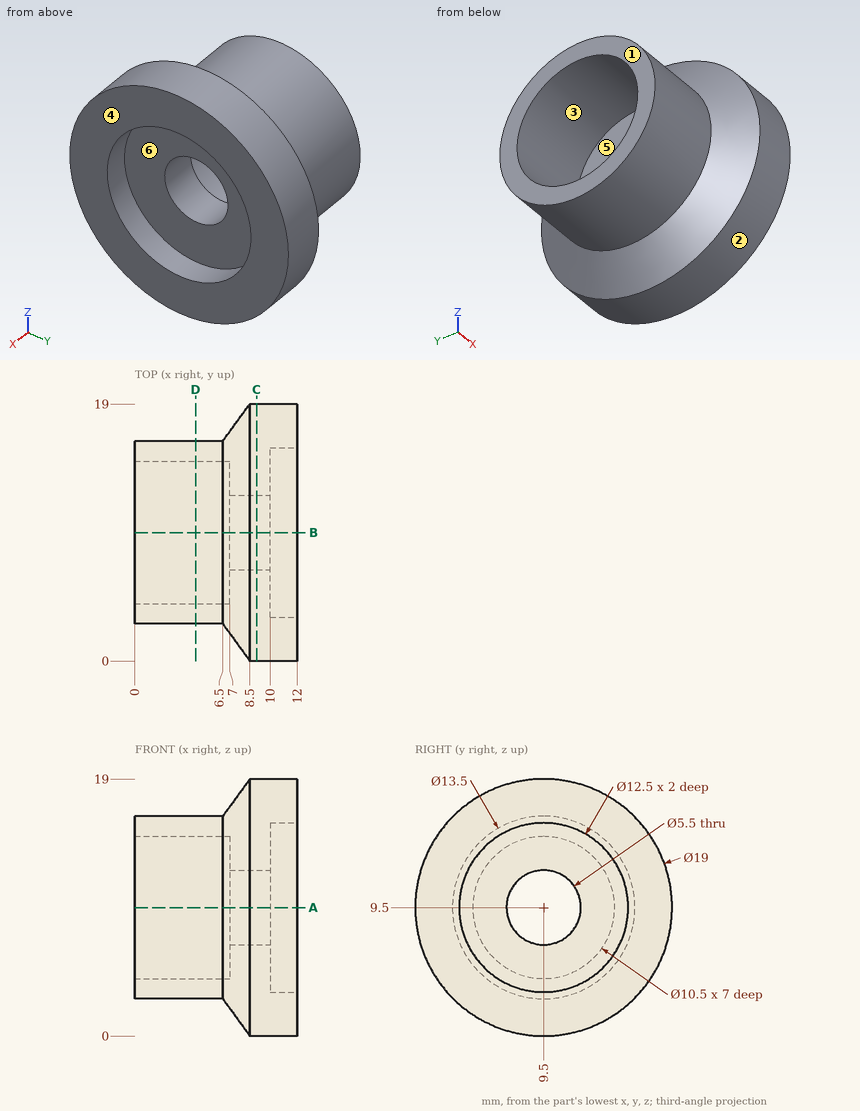
Verification items for this drawing (mm, ordinates from the low corner). A direction names the side the tool comes from. Give positions to 0.01 mm unless a question says otherwise; leave off trailing zeros. Loops run counter-clockwise (first coordinate to the right, second up) from the corner with the lowest first, then second, coordinate; pieces in that order, holes last. Notation, with made-up numbers: M 56.25,1.25 L 91.25,1.25 A22 ccw 91.25,9.25 Z; hole C -5.75,-33 d9. An arc over 180 degrees is marked long. Answer as a JSON object with one key per item and string values. Group by question number.
Q1. Go/stop test with flat-tipped pins: P1, Ø7.5, axis at y = 9.5, z = 9.5, coming from the -X side; P2, Ø5, axis at x = 3.5, y = 12, coming from the -Z side; P3, Ø4, axis at y = 7.5, z = 7.5, coming from the +X side. Record where each tip stops, or that it passes through.
Q2. Release check for a two-part mould opening along Y. For the marked faces 1, 2 and 3 record: released by +Y, released by -Y, zero draft, split by the parting line, or undercut.
Q3. Cross-section at D-D on x = 4.5. Record the cut outline in (y, z).
Q4. Cross-section at A-A on z = 9.5. Record the cut outline in (x, y), then the cut area to 4 significant figures.
Q5. Material ranges on line 1 along Y through (x, z) = (9.1, 9.5); line 2 along Y through (x, z) = (10.5, 9.75) (3 decimals); line 3 along Z through (x, y) = (3.25, 9.5), recorded low to high. Write a range as [from, to].
Q6. Access from +Z, -Z, +X, -X, +Y, -Y to the whole of each face (thin tool, end or side, straight path). Record for the marked faces 4, 5 and 6.
Q7. Cross-section at C-C on x = 9. Record the cut outline in (y, z).
Evaluation:
{
 "1": {"P1": "stops at x = 7", "P2": "stops at z = 2.75", "P3": "stops at x = 10"},
 "2": {"face 1": "zero draft", "face 2": "split by the parting line", "face 3": "undercut"},
 "3": {"outline": "C 9.5,9.5 d13.5; hole C 9.5,9.5 d10.5"},
 "4": {"outline": "M 0,2.75 L 6.5,2.75 L 8.5,0 L 12,0 L 12,3.25 L 10,3.25 L 10,6.75 L 7,6.75 L 7,4.25 L 0,4.25 Z; M 0,14.75 L 7,14.75 L 7,12.25 L 10,12.25 L 10,15.75 L 12,15.75 L 12,19 L 8.5,19 L 6.5,16.25 L 0,16.25 Z", "area": "71.75 mm2"},
 "5": {"line 1": "y = [0, 6.75], [12.25, 19]", "line 2": "y = [0.003, 3.255], [15.745, 18.997]", "line 3": "z = [2.75, 4.25], [14.75, 16.25]"},
 "6": {"face 4": "+Z, -Z, +X, +Y, -Y", "face 5": "-X", "face 6": "+X"},
 "7": {"outline": "C 9.5,9.5 d19; hole C 9.5,9.5 d5.5"}
}
